Source: CAD feature listing. Evaluate the final solid. Frame: model axes, mm. A direction names the side the tool comes from. Coordinates: 2 decimals unless noted, no trailing zeros. Order: outer loops, then holes, each group sorted by start corner. A loop starts at its lowest first (then second) coordinate and runs counter-clockwise, first axis right, second up. Notation, with made-up numbers: (18.25, 25) - (55.25, 25) arc R18 cw to (55.25, 57) - close; hole circle Ø10 at (-3, -32). An arc over 180 degrees is marked (long way). One line per question, with ' | ' between items. Start each with the question number.
(1) Section C-C (x = 0). Return the cut outline in (y, z).
(2) Section B-B (y = -11). Return the cut outline in (x, z).
(3) Draft query along Z for faces 4 (the cylindrical face through (-14.1, -7.4, -0.7)), 5 (the cylindrical face through (-0.28, -0.57, -0.6)), 6 (the cylindrical face through (-8.39, -0.74, -39.98)). Return one class per face: +Z half, -Z half, draft (parallel to the pull), parting line (faces both ways), or undercut.
(4) Section D-D (z = -6.5). Return the cut outline in (x, y).
(5) Line query: line 1 along X through (y, z) = (-0.85, -6.5); line 2 along X through (y, z) = (-0.7, -38.5); line 3 along Z through (x, y) = (9, -0.4). Output: solid intervals per line, ascending.
(6) Access query for faces 1 (the flat face through (-6.25, -1, -22)), 2 (the cylindrical face through (9.1, -23.5, -0.8)), 3 (the flat face through (0, -30, -1)). Directions: +Z, -Z, +X, -X, +Y, -Y. A direction counts if a zero-diameter tool reaches every point of the face in a straight line with its end or side. Return the directions, or none.
(7) Contact query for flat-ended pins moving along their axis: P1, Ø2, axis at x = -14.5, y = -12, coming from the +Z side; P2, Ø1.5, axis at x = 15.5, z = -41.5, coming from the -Y side; P3, Ø14, axis at x = 4, y = -16.5, coming from the -Z side. Output: stop coordinate, or through.
(8) Section A-A (z = -27.5). Return the cut outline in (x, y), then the cut area to 4 significant figures.
from build123d import *

# Parameters (mm, degrees)
BOSS_EXTRUDE1_DEPTH           = 30
SKETCH2_W                     = 28.5
SKETCH2_H                     = 28.5
CUT_EXTRUDE1_DEPTH            = 71.710678119
CUT_EXTRUDE2_REACH            = 63.644
CUT_EXTRUDE3_REACH            = 63.644
CUT_EXTRUDE4_REACH            = 63.644
CUT_EXTRUDE5_DEPTH            = 61.928236475
CUT_EXTRUDE6_DEPTH            = 61.433848132
SKETCH8_W                     = 1.601710745
SKETCH8_H                     = 1.5
M3_CLEARANCE_HOLE1_AT_2_COUNT = 2
M3_CLEARANCE_HOLE1_AT_2_PITCH = 18
M3_CLEARANCE_HOLE1_AT_3_COUNT = 2
M3_CLEARANCE_HOLE1_AT_3_PITCH = 32
M3_CLEARANCE_HOLE1_AT_4_COUNT = 2
M3_CLEARANCE_HOLE1_AT_4_PITCH = 36.715119501
M3_CLEARANCE_HOLE1_AT_5_COUNT = 2
M3_CLEARANCE_HOLE1_AT_5_PITCH = 23.858424089
M3_CLEARANCE_HOLE1_AT_6_COUNT = 2
M3_CLEARANCE_HOLE1_AT_6_PITCH = 32.272967016
FILLET1_R                     = 0.5
FILLET2_R                     = 2
FILLET3_R                     = 4
CUT_EXTRUDE7_DEPTH            = 28.5
SKETCH11_R                    = 1.801810181
CUT_EXTRUDE8_DEPTH            = 62.64414003


with BuildPart() as part:
    # Sketch1 → Boss-Extrude1 (new body)
    with BuildSketch(Plane.XZ.offset(30)):
        with BuildLine():
            Line((20, 0), (-20, 0))
            Line((-20, 0), (-20, -30))
            ThreePointArc((-20, -30), (0, -50), (20, -30))
            Line((20, -30), (20, 0))
        make_face()
    extrude(amount=-BOSS_EXTRUDE1_DEPTH)

    # Sketch2 → Cut-Extrude1 (cut, through all)
    with BuildSketch(Plane(origin=(20, 0, 0), x_dir=(0, 0, -1), z_dir=(1, 0, 0))):
        with Locations((15.75, -15.75)):
            Rectangle(SKETCH2_W, SKETCH2_H)
    extrude(amount=-CUT_EXTRUDE1_DEPTH, mode=Mode.SUBTRACT)

    # Sketch3 → Cut-Extrude2 (cut, up to next)
    with BuildSketch(Plane.XY, mode=Mode.PRIVATE) as cut_extrude2_sk1:
        with BuildLine():
            Line((16.2, -23.5), (16.2, -9.5))
            ThreePointArc((16.2, -9.5), (14.1, -7.4), (12, -9.5))
            Line((12, -9.5), (12, -23.5))
            ThreePointArc((12, -23.5), (14.1, -25.6), (16.2, -23.5))
        make_face()
    cut_extrude2_tool1 = extrude(cut_extrude2_sk1.sketch, amount=-CUT_EXTRUDE2_REACH, mode=Mode.PRIVATE) & part.part
    add(cut_extrude2_tool1.solids().sort_by_distance((14.1, -16.5, 0))[0], mode=Mode.SUBTRACT)

    # Sketch4 → Cut-Extrude3 (cut, up to next)
    with BuildSketch(Plane.XY, mode=Mode.PRIVATE) as cut_extrude3_sk1:
        with BuildLine():
            Line((-16.2, -9.5), (-16.2, -23.5))
            ThreePointArc((-16.2, -23.5), (-14.1, -25.6), (-12, -23.5))
            Line((-12, -23.5), (-12, -9.5))
            ThreePointArc((-12, -9.5), (-14.1, -7.4), (-16.2, -9.5))
        make_face()
    cut_extrude3_tool1 = extrude(cut_extrude3_sk1.sketch, amount=-CUT_EXTRUDE3_REACH, mode=Mode.PRIVATE) & part.part
    add(cut_extrude3_tool1.solids().sort_by_distance((-14.1, -16.5, 0))[0], mode=Mode.SUBTRACT)

    # Sketch5 → Cut-Extrude4 (cut, up to next)
    with BuildSketch(Plane.XY, mode=Mode.PRIVATE) as cut_extrude4_sk1:
        with BuildLine():
            Line((-6.981600402, -11.599919392), (6.981600402, -11.599919392))
            ThreePointArc((6.981600402, -11.599919392), (9.099979848, -9.509199887), (7, -7.4))
            Line((7, -7.4), (-7, -7.4))
            ThreePointArc((-7, -7.4), (-9.099979848, -9.509199887), (-6.981600402, -11.599919392))
        make_face()
    cut_extrude4_tool1 = extrude(cut_extrude4_sk1.sketch, amount=-CUT_EXTRUDE4_REACH, mode=Mode.PRIVATE) & part.part
    add(cut_extrude4_tool1.solids().sort_by_distance((0, -9.499967, 0))[0], mode=Mode.SUBTRACT)

    # Sketch6 → Cut-Extrude5 (cut, through all)
    with BuildSketch(Plane.XZ.offset(1.5)):
        with BuildLine():
            Line((6.25, -30), (6.25, -15))
            ThreePointArc((6.25, -15), (0, -8.75), (-6.25, -15))
            Line((-6.25, -15), (-6.25, -30))
            ThreePointArc((-6.25, -30), (0, -36.25), (6.25, -30))
        make_face()
    extrude(amount=-CUT_EXTRUDE5_DEPTH, mode=Mode.SUBTRACT)

    # Sketch7 → Cut-Extrude6 (cut, through all)
    with BuildSketch(Plane(origin=(0, 0, -1.5), x_dir=(-1, 0, 0), z_dir=(0, 0, -1))):
        with BuildLine():
            Line((-7, -25.6), (7, -25.6))
            ThreePointArc((7, -25.6), (9.1, -23.5), (7, -21.4))
            Line((7, -21.4), (-7, -21.4))
            ThreePointArc((-7, -21.4), (-9.1, -23.5), (-7, -25.6))
        make_face()
    extrude(amount=-CUT_EXTRUDE6_DEPTH, mode=Mode.SUBTRACT)

    # Sketch8 → M3 Clearance Hole1 (revolve, cut)
    with BuildSketch(Plane(origin=(-9, -1.5, -6.5), x_dir=(0, 0, -1), z_dir=(1, 0, 0))):
        with Locations((0.800855373, 0.75)):
            Rectangle(SKETCH8_W, SKETCH8_H)
    m3_clearance_hole1 = revolve(axis=Axis((-9, -7.85, -6.5), (0, 1, 0)), mode=Mode.SUBTRACT)

    # M3 Clearance Hole1 at 2: M3 Clearance Hole1 ×2
    with Locations(*[(i * M3_CLEARANCE_HOLE1_AT_2_PITCH, 0, 0) for i in range(1, M3_CLEARANCE_HOLE1_AT_2_COUNT)]):
        add(m3_clearance_hole1, mode=Mode.SUBTRACT)

    # M3 Clearance Hole1 at 3: M3 Clearance Hole1 ×2
    with Locations(*[(0, 0, -i * M3_CLEARANCE_HOLE1_AT_3_PITCH) for i in range(1, M3_CLEARANCE_HOLE1_AT_3_COUNT)]):
        add(m3_clearance_hole1, mode=Mode.SUBTRACT)

    # M3 Clearance Hole1 at 4: M3 Clearance Hole1 ×2
    with Locations(*[Vector(0.4902612396325592, 0, -0.8715755371245493) * (i * M3_CLEARANCE_HOLE1_AT_4_PITCH) for i in range(1, M3_CLEARANCE_HOLE1_AT_4_COUNT)]):
        add(m3_clearance_hole1, mode=Mode.SUBTRACT)

    # M3 Clearance Hole1 at 5: M3 Clearance Hole1 ×2
    with Locations(*[Vector(-0.17268533682984544, 0, -0.9849770425974216) * (i * M3_CLEARANCE_HOLE1_AT_5_PITCH) for i in range(1, M3_CLEARANCE_HOLE1_AT_5_COUNT)]):
        add(m3_clearance_hole1, mode=Mode.SUBTRACT)

    # M3 Clearance Hole1 at 6: M3 Clearance Hole1 ×2
    with Locations(*[Vector(0.6854033590776325, 0, -0.7281636048067069) * (i * M3_CLEARANCE_HOLE1_AT_6_PITCH) for i in range(1, M3_CLEARANCE_HOLE1_AT_6_COUNT)]):
        add(m3_clearance_hole1, mode=Mode.SUBTRACT)

    # Fillet1
    fillet1_edges = [part.edges().sort_by_distance(p)[0] for p in [
        (0, -1.5, -1.5),
    ]]
    fillet(fillet1_edges, radius=FILLET1_R)

    # Fillet2
    fillet2_edges = [part.edges().sort_by_distance(p)[0] for p in [
        (0, 0, 0),
    ]]
    fillet(fillet2_edges, radius=FILLET2_R)

    # Fillet3
    fillet3_edges = [part.edges().sort_by_distance(p)[0] for p in [
        (20, -30, -0.75),
        (-20, -30, -0.75),
    ]]
    fillet(fillet3_edges, radius=FILLET3_R)

    # Sketch10 → Cut-Extrude7 (cut)
    with BuildSketch(Plane.XZ.offset(30)):
        with BuildLine():
            Line((-20, -30), (20, -30))
            ThreePointArc((20, -30), (0, -50), (-20, -30))
        make_face()
    extrude(amount=-CUT_EXTRUDE7_DEPTH, mode=Mode.SUBTRACT)

    # Sketch11 → Cut-Extrude8 (cut, through all)
    with BuildSketch(Plane(origin=(0, 0, 0), x_dir=(1, 0, 0), z_dir=(0, 1, 0))):
        with Locations(Location((-15.73061053, 23.534870495, 0), (0, 0, 270))):
            Circle(SKETCH11_R)
        with Locations(Location((15.251209648, 22.473339956, 0), (0, 0, 270))):
            Circle(SKETCH11_R)
    extrude(amount=-CUT_EXTRUDE8_DEPTH, mode=Mode.SUBTRACT)


solid = part.part
Response values:
1) outline: (-30, -1.5) - (-25.6, -1.5) - (-25.6, 0) - (-30, 0) - close; (-21.4, -1.5) - (-11.6, -1.5) - (-11.6, 0) - (-21.4, 0) - close; (-7.4, -1.5) - (-2, -1.5) arc R0.5 cw to (-1.5, -2) - (-1.5, -8.75) - (0, -8.75) - (0, -2) arc R2 ccw to (-2, 0) - (-7.4, 0) - close; (-1.5, -50) - (0, -50) - (0, -36.25) - (-1.5, -36.25) - close
2) outline: (-20, -1.5) - (-16.2, -1.5) - (-16.2, 0) - (-20, 0) - close; (-12, -1.5) - (-8.47, -1.5) - (-8.47, 0) - (-12, 0) - close; (8.47, -1.5) - (12, -1.5) - (12, 0) - (8.47, 0) - close; (16.2, -1.5) - (20, -1.5) - (20, 0) - (16.2, 0) - close
3) face 4: draft | face 5: +Z half | face 6: undercut
4) outline: (-20, -1.5) - (-10.6, -1.5) - (-10.6, 0) - (-20, 0) - close; (-7.4, -1.5) - (7.4, -1.5) - (7.4, 0) - (-7.4, 0) - close; (10.6, -1.5) - (20, -1.5) - (20, 0) - (10.6, 0) - close
5) line 1: x = -20 to -10.6, -7.4 to 7.4, 10.6 to 20 | line 2: x = -18.1 to -10.6, -7.4 to 7.4, 10.6 to 18.1 | line 3: z = -47.86 to -40.1, -36.9 to -8.1, -4.9 to -0.8
6) face 1: +Y, -Y | face 2: +Z, -Z | face 3: +Z, -Z, +X, -X, -Y
7) P1: passes through | P2: stops at y = -1.5 | P3: stops at z = -1.5
8) outline: (-20, -1.5) - (-6.25, -1.5) - (-6.25, 0) - (-20, 0) - close; (6.25, -1.5) - (20, -1.5) - (20, 0) - (6.25, 0) - close | area: 41.25 mm²
